Geometry: see drawing. Coordinates: mm, zero at the bounding-box minimum. A direction names the side the tool comes from. Round coordinates to 2 decimals unless told otherwise and drop trailing zeros. Loops run counter-clockwise (first coordinate to the right, second up) from the corner with the lowest first, then second, coordinate; pieces in that order, holes last.
(1) Section A-A, the plane y = 6.5. Return the cut outline in (x, z).
(2) Mould query, pull axis Z, two halves, no side actions, for the marked faces 1, 2 and 3. Classes: pulls with the +Z half, pulls with the -Z half, needs draft (parallel to the pull), parting line crosses it, or undercut.
(3) Set-up query: the marked faces 4 and 5. Return all of +Z, -Z, +X, -X, +Y, -Y with unobstructed straight access to the full face (end or side cutting, diameter ignored); none if empty.
(4) First-contact query: pin 1 Ø3 at (y, z) = (9, 8) entering from +X; pin 2 Ø5.5 at (x, z) = (10, 10) entering from -Y; pin 3 Ø1 at (y, z) = (13.5, 4.5) entering from -X. Flat tips, straight axial feed; report the tip coordinate or a pass-through.
(5) Material intervals for probe 1 along Z at (x, y) = (10, 2.3); probe 2 along Z at (x, y) = (12.5, 4.5); probe 3 along X at (y, z) = (5.25, 18), sorted ascending.
(6) Section B-B, the plane y = 13. Return the cut outline in (x, z).
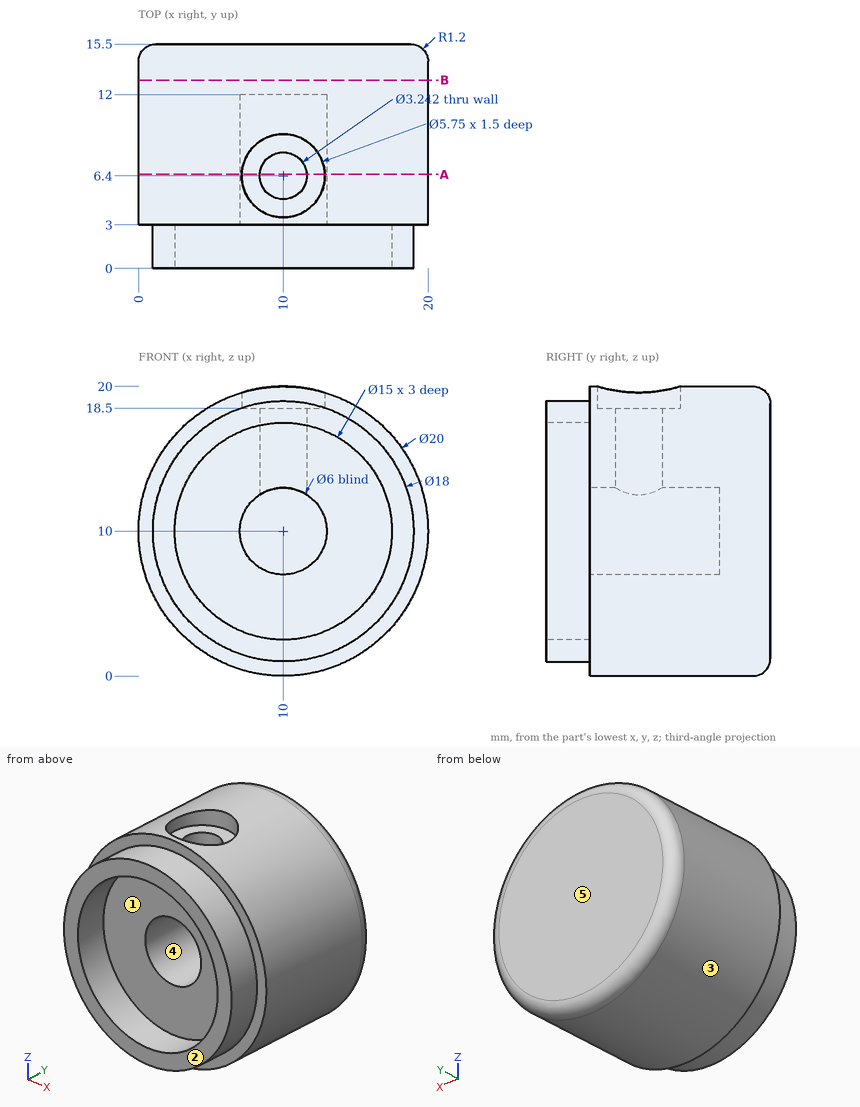
Output values:
1. outline: (7.13, 18.5) - (7.13, 19.58) arc R10 ccw (long way) to (12.87, 19.58) - (12.87, 18.5) - (11.62, 18.5) - (11.62, 12.53) arc R3 cw (long way) to (8.38, 12.53) - (8.38, 18.5) - close
2. face 1: undercut
2. face 2: needs draft
2. face 3: parting line crosses it
3. face 4: -Y
3. face 5: +Z, -Z, +X, -X, +Y
4. pin 1: stops at x = 19.99
4. pin 2: stops at y = 12
4. pin 3: stops at x = 1.34
5. probe 1: z = 1 to 2.5, 17.5 to 19
5. probe 2: z = 0.32 to 8.34, 11.66 to 19.68
5. probe 3: x = 4 to 8.86, 11.14 to 16
6. outline: circle Ø20 at (10, 10)
